Here's how the part is built. I have some questions about the finished solid (model axes, mm). Face numbers are marked on the shaded views. A direction names the side the tool comes from. Coordinates: 2 decimals unless noted, no trailing zeros. Write each loop counter-clockwise with the first axis right and the second up, starting at its lowest first coordinate (ties: lowest second). Pieces come first, ordered by that corner, then holes.
Autodesk Inventor part; units mm, degrees
ref_plane "Work Plane1" through (-30, 0, 0) normal (1, 0, 0) x (0, 0, -1)
ref_plane "YZ Plane" through (0, 0, 0) normal (1, 0, 0) x (0, 1, 0)
ref_plane "XZ Plane" through (0, 0, 0) normal (0, 1, 0) x (-1, 0, 0)
sketch "Sketch1" plane through (0, 0, 0) normal (1, 0, 0) x (0, 1, 0)
  circle A0 centre (0, 0) radius 500
  circle A1 centre (0, 0) radius 625
  dimension "d0" = 1000
  dimension "d1" = 1250
extrude "Extrusion1" add sketch "Sketch1" against normal blind 210
sketch "Sketch2" plane through (0, 0, 0) normal (1, 0, 0) x (0, 0, -1)
  circle A0 centre (0, 0) radius 650
  circle A1 centre (0, 0) radius 625
  dimension "d4" = 1300
sketch "Sketch3" plane through (-210, 0, 0) normal (-1, 0, 0) x (0, 0, 1)
  circle A0 centre (0, 0) radius 650
  circle A1 centre (0, 0) radius 625
  dimension "d5" = 1300
extrude "Extrusion2" add sketch "Sketch3" against normal blind 30
extrude "Extrusion3" add sketch "Sketch2" against normal blind 30
ref_plane "Work Plane1" through (-30, 0, 0) normal (1, 0, 0) x (0, 0, -1)
sketch "Sketch4" plane through (-30, 0, 0) normal (1, 0, 0) x (0, 0, -1)
  circle A0 centre (0, 0) radius 125
  dimension "d11" = 250
extrude "Extrusion4" add sketch "Sketch4" against normal blind 150
sketch "Sketch5" plane through (-30, 0, 0) normal (1, 0, 0) x (0, 0, -1)
  line L0 (0, 0) -> (469.0204, 0) construction
  line L1 (0, 0) -> (-234.5102, 406.1836) construction
  line L2 (0, 0) -> (-234.5102, -406.1836) construction
  line L3 (0, -910) -> (0, 910)
  line L4 (520.2054, 50) -> (0, 50)
  line L5 (0, 50) -> (0, -50)
  line L6 (0, -50) -> (520.2054, -50)
  line L7 (520.2054, -50) -> (520.2054, 50)
  line L8 (-216.8015, 475.5111) -> (-303.404, 425.5111)
  line L9 (43.3013, 25) -> (-216.8015, 475.5111)
  line L10 (-303.404, 425.5111) -> (-43.3013, -25)
  line L11 (-43.3013, -25) -> (43.3013, 25)
  line L12 (-303.404, -425.5111) -> (-216.8015, -475.5111)
  line L13 (-43.3013, 25) -> (-303.404, -425.5111)
  line L14 (-216.8015, -475.5111) -> (43.3013, -25)
  line L15 (43.3013, -25) -> (-43.3013, 25)
  point P0 (234.5102, 0)
  point P1 (0, 0)
  point P2 (0, 0)
  point P3 (0, 0)
  point P4 (28.8675, 50)
  point P5 (-57.735, 0)
  point P6 (28.8675, -50)
  dimension "d16" = 360
  dimension "d18" = 90
  dimension "d19" = 100
  dimension "d20" = 50
  dimension "d21" = 0
  dimension "d24" = 360
extrude "Extrusion5" add sketch "Sketch5" against normal blind 150
sketch "Sketch6" plane through (-30, 0, 0) normal (1, 0, 0) x (0, 0, -1)
  circle A0 centre (0, 0) radius 30
  dimension "d28" = 60
extrude "Extrusion6" cut sketch "Sketch6" against normal through all
sketch "Sketch7" plane through (-30, 0, 0) normal (1, 0, 0) x (0, 0, -1)
  line L0 (33, 4) -> (28, 4)
  line L1 (28, 4) -> (28, -4)
  line L2 (28, -4) -> (33, -4)
  line L3 (33, -4) -> (33, 4)
  line L4 (910, 0) -> (-910, 0)
  circle A0 centre (0, 0) radius 30
  point P0 (33, 0)
  dimension "d31" = 8
  dimension "d32" = 5
  dimension "d33" = 4
  dimension "d34" = 33
extrude "Extrusion7" cut sketch "Sketch7" against normal through all contours L3 L4 A0 L0 | A0 L4 L1 L0 | L3 L2 A0 L4 | A0 L2 L1 L4 picked at (28.627, 2.2237) picked at (28.627, -2.2237)
properties part number "Wheel1"
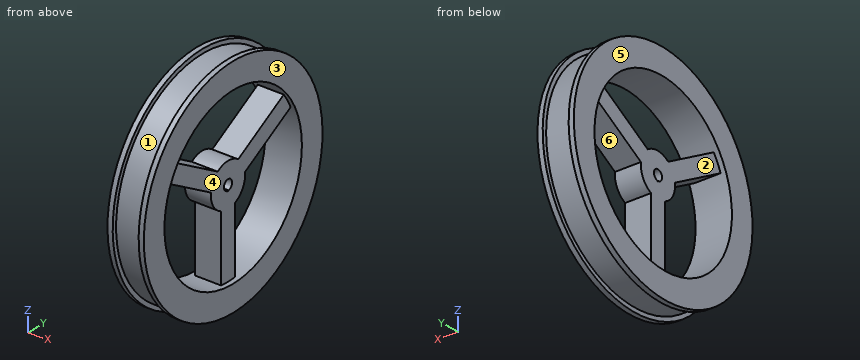
1) Imagine slicing it at A-A on z = -188.5. Please give me the cut outline in (x, y).
Values follow:
outline: (-210, -622.07) - (-180, -622.07) - (-180, -595.9) - (-30, -595.9) - (-30, -622.07) - (0, -622.07) - (0, -463.11) - (-210, -463.11) - close; (-210, 463.11) - (0, 463.11) - (0, 622.07) - (-30, 622.07) - (-30, 595.9) - (-180, 595.9) - (-180, 622.07) - (-210, 622.07) - close; (-180, -50) - (-30, -50) - (-30, 50) - (-180, 50) - close
2) Will these pins go through, and if not, where does the flat tip stop? pin 1 (3 mm diameter, centred on x = -73, y = 61, fed in from -Z); pin 2 (4 mm diameter, centred on x = -109, y = 458, fed in from +Z); pin 3 (5 mm diameter, centred on x = -135.5, z = 452, fed in from -Y).
Values follow:
pin 1: stops at z = -622.16
pin 2: stops at z = 427.42
pin 3: stops at y = -434.25
3) Imagine slicing it at C-C on z = 449. Please give me the cut outline in (x, y), then the cut area to 3 significant figures.
Values follow:
outline: (-210, -470) - (-180, -470) - (-180, -434.77) - (-30, -434.77) - (-30, -470) - (0, -470) - (0, -220) - (-210, -220) - close; (-210, 220) - (0, 220) - (0, 470) - (-30, 470) - (-30, 434.77) - (-180, 434.77) - (-180, 470) - (-210, 470) - close
area: 94,400 mm2
4) I need wall thicknesses on probe 1 along Z at (x, y) = (-151, 0); probe 2 along X at (y, z) = (-447.5, 469.5); probe 3 along Y at (x, z) = (-91.5, -332). Which ranges of each line are inside material? Lowest first, please.
Values follow:
probe 1: z = -625 to -33, 30 to 125, 500 to 625
probe 2: x = -210 to -180, -30 to 0
probe 3: y = -529.53 to -373.87, -50 to 50, 373.87 to 529.53
5) We'd pull the mould along Y, two halves only. Please class the marked faces 1, 2 and 3: pulls with the +Y half, pulls with the -Y half, needs draft (parallel to the pull), parting line crosses it, or undercut.
Values follow:
face 1: parting line crosses it
face 2: undercut
face 3: needs draft
6) Imagine slicing it at D-D on y = 211.5. Please give me the cut outline in (x, z), then the cut area to 3 significant figures.
Values follow:
outline: (-210, -614.63) - (-180, -614.63) - (-180, -588.13) - (-30, -588.13) - (-30, -614.63) - (0, -614.63) - (0, -453.06) - (-210, -453.06) - close; (-210, 453.06) - (0, 453.06) - (0, 614.63) - (-30, 614.63) - (-30, 588.13) - (-180, 588.13) - (-180, 614.63) - (-210, 614.63) - close; (-180, 64.37) - (-30, 64.37) - (-30, 179.84) - (-180, 179.84) - close
area: 77,200 mm2
7) Imagine slicing it at B-B on x = -99. Please give me the cut outline in (y, z), then the cut area to 3 significant figures.
Values follow:
outline: circle Ø1250 at (0, 0); hole (-455.84, 205.45) arc R500 ccw to (-50, -497.49) - (-50, -114.56) arc R125 cw to (-124.22, 13.98) - close; hole (-405.84, 292.05) - (-74.22, 100.58) arc R125 cw to (74.22, 100.58) - (405.84, 292.05) arc R500 ccw to start; hole (-4, -33) - (4, -33) - (4, -29.73) arc R30 ccw (long way) to (-4, -29.73) - close; hole (50, -497.49) arc R500 ccw to (455.84, 205.45) - (124.22, 13.98) arc R125 cw to (50, -114.56) - close
area: 601,000 mm2
8) On a 3-axis mill with a long thin cutter (end or side, diameter ignored), from which of +Z, -Z, +X, -X, +Y, -Y can I reach the whole of each face in a straight line? I mean the marked faces 4, 5 and 6. Say none if no direction works.
Values follow:
face 4: +X
face 5: +Z, -Z, -X, +Y, -Y
face 6: +X, -X
